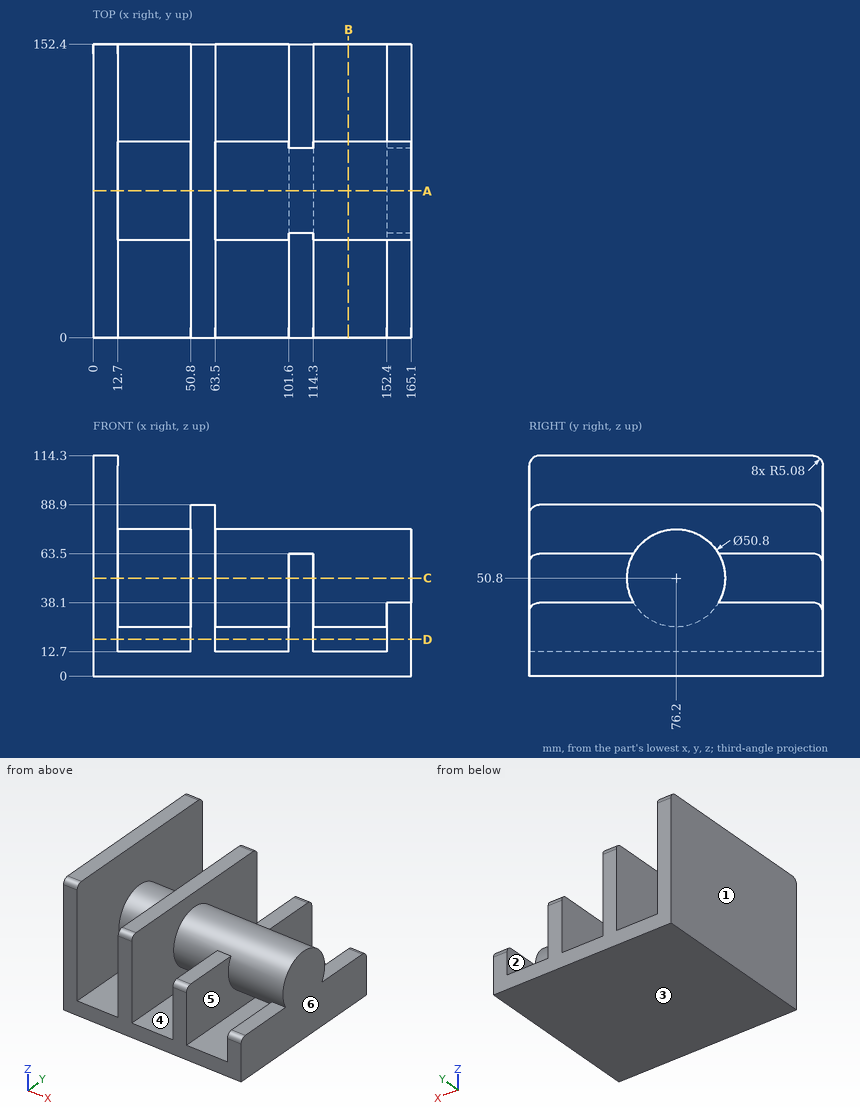
Source: three-view drawing plus pictorial views. Frame: mm from the lowest corner of the part. A direction names the side the tool comes from. Round coordinates to 2 decimals unless told otherwise and drop trailing zeros. Loops run counter-clockwise (first coordinate to the right, second up) from the corner with the lowest first, then second, coordinate; pieces in that order, holes last. Notation, with made-up numbers: M 46.5,67.5 L 55.5,67.5 A14 cw 55.5,91.5 Z; hole C -31.5,-36.75 d4. An arc over 180 degrees is marked long. Put each result on its own line as item: value. Start each with the question number.
(1) Section query C-C (z = 50.8). Return loops of the section in (x, y), then the cut area to 3 significant figures.
(2) Contact query for flat-ended pins moving along their axis: pin 1 Ø10 at (x, y) = (158, 25.5) entering from +Z; pin 2 Ø2 at (y, z) = (22.5, 47) entering from -X; pin 3 Ø10 at (x, z) = (31.5, 68) entering from -Y; pin 4 Ø8 at (x, z) = (87, 36.5) entering from +Y. Output: stop coordinate, or through.
(3) Material intervals for line 1 along X through (y, z) = (27.5, 35); line 2 along X through (y, z) = (23, 48); line 3 along X through (y, z) = (116, 86), sorted ascending. Write a range as [from, to].
(4) Section query A-A (y = 76.2). Return loops of the section in (x, z), then the cut area to 3 significant figures.
(5) Section query B-B (x = 132.5). Return loops of the section in (y, z), then the cut area to 3 significant figures.
(6) Draft query along X for the marked faces 1, 2 and 3. Return one class per face: +X half, -X half, draft (parallel to the pull), parting line (faces both ways), or undercut.
(7) Section query D-D (z = 19). Return loops of the section in (x, y).
(8) Set-up query: the marked faces 4, 5 and 6. Return all of +Z, -Z, +X, -X, +Y, -Y with unobstructed straight access to the full face (end or side cutting, diameter ignored); none if empty.
Findings below:
1. outline: M 0,0 L 12.7,0 L 12.7,50.8 L 50.8,50.8 L 50.8,0 L 63.5,0 L 63.5,50.8 L 101.6,50.8 L 101.6,0 L 114.3,0 L 114.3,50.8 L 165.1,50.8 L 165.1,101.6 L 114.3,101.6 L 114.3,152.4 L 101.6,152.4 L 101.6,101.6 L 63.5,101.6 L 63.5,152.4 L 50.8,152.4 L 50.8,101.6 L 12.7,101.6 L 12.7,152.4 L 0,152.4 Z
1. area: 12,300 mm2
2. pin 1: stops at z = 38.1
2. pin 2: stops at x = 0
2. pin 3: stops at y = 53.92
2. pin 4: stops at y = 99.42
3. line 1: x = [0, 12.7], [50.8, 63.5], [101.6, 114.3], [152.4, 165.1]
3. line 2: x = [0, 12.7], [50.8, 63.5], [101.6, 114.3]
3. line 3: x = [0, 12.7], [50.8, 63.5]
4. outline: M 0,0 L 165.1,0 L 165.1,76.2 L 63.5,76.2 L 63.5,88.9 L 50.8,88.9 L 50.8,76.2 L 12.7,76.2 L 12.7,114.3 L 0,114.3 Z; hole M 12.7,12.7 L 50.8,12.7 L 50.8,25.4 L 12.7,25.4 Z; hole M 63.5,12.7 L 101.6,12.7 L 101.6,25.4 L 63.5,25.4 Z; hole M 114.3,12.7 L 152.4,12.7 L 152.4,25.4 L 114.3,25.4 Z
4. area: 11,800 mm2
5. outline: M 0,0 L 152.4,0 L 152.4,12.7 L 0,12.7 Z; C 76.2,50.8 d50.8
5. area: 3,960 mm2
6. face 1: -X half
6. face 2: undercut
6. face 3: draft
7. outline: M 0,0 L 12.7,0 L 12.7,152.4 L 0,152.4 Z; M 50.8,0 L 63.5,0 L 63.5,152.4 L 50.8,152.4 Z; M 101.6,0 L 114.3,0 L 114.3,152.4 L 101.6,152.4 Z; M 152.4,0 L 165.1,0 L 165.1,152.4 L 152.4,152.4 Z
8. face 4: +Y, -Y
8. face 5: none
8. face 6: +Z, -Z, +X, +Y, -Y
